CAD build for the part. Positions are in the model's coordinates, mm. A direction names the side the tool comes from. Give positions to 0.01 mm unless a question says otherwise; leave off trailing zeros. Write each loop counter-clockwise with the first axis right and the second up, starting at its lowest first coordinate (ties: lowest second). Pieces come first, ordered by that corner, then holes. Notation, with made-up numbers: (44, -31) - (62, -31) arc R21 ccw to (62, -15) - close; hole circle Ø1 at (66.5, 24). An arc over 180 degrees is marked (long way). Answer as a JSON object with one key per item and string values.
from build123d import *

# Parameters (mm, degrees)
SKETCH_1_W          = 41
SKETCH_1_H          = 64
EXTRUDE_1_DEPTH     = 4
SKETCH_2_R          = 1.75
CUT_EXTRUDE_1_DEPTH = 3
FILLET_1_R          = 2
CHAMFER_2_SIZE      = 1
CHAMFER_1_SIZE      = 2
CHAMFER_3_SIZE      = 0.5


with BuildPart() as part:
    # Эскиз1 → Бобышка-Вытянуть1 (new body)
    with BuildSketch(Plane(origin=(0, 0, 0), x_dir=(1, 0, 0), z_dir=(0, 1, 0))):
        Rectangle(SKETCH_1_W, SKETCH_1_H)
    extrude(amount=EXTRUDE_1_DEPTH)

    # Эскиз2 → Вырез-Вытянуть1 (cut)
    with BuildSketch(Plane(origin=(0, 4, 0), x_dir=(1, 0, 0), z_dir=(0, 1, 0))):
        with Locations(Location((16, 18, 0), (0, 0, 270))):
            Circle(SKETCH_2_R)
        with Locations(Location((16, -28, 0), (0, 0, 90))):
            Circle(SKETCH_2_R)
        with Locations(Location((-16, 18, 0), (0, 0, 90))):
            Circle(SKETCH_2_R)
        with Locations(Location((-16, -28, 0), (0, 0, 270))):
            Circle(SKETCH_2_R)
    extrude(amount=-CUT_EXTRUDE_1_DEPTH, mode=Mode.SUBTRACT)

    # Скругление1
    fillet_1_edges = [part.edges().sort_by_distance(p)[0] for p in [
        (20.5, 2, 32),
        (-20.5, 2, 32),
        (-20.5, 2, -32),
        (20.5, 2, -32),
    ]]
    fillet(fillet_1_edges, radius=FILLET_1_R)

    # Фаска2
    chamfer_2_edges = [part.edges().sort_by_distance(p)[0] for p in [
        (0, 4, -32),
        (20.5, 4, 0),
        (-20.5, 4, 0),
        (0, 4, 32),
        (19.914213562, 4, 31.414213562),
        (-19.914213562, 4, 31.414213562),
        (-19.914213562, 4, -31.414213562),
        (19.914213562, 4, -31.414213562),
    ]]
    chamfer(chamfer_2_edges, length=CHAMFER_2_SIZE)

    # Фаска1
    # the kernel refuses this chamfer: 2 mm, written as the material it takes off along each edge
    with BuildSketch(Plane(origin=(-16, 4, -18), x_dir=(0, 0, -1), z_dir=(1, 0, 0))) as chamfer_1_piece_1:
        Polygon((1.75 + CHAMFER_1_SIZE, 0), (1.75, -CHAMFER_1_SIZE), (1.75, 0), align=None)
    revolve(axis=Axis((-16, 4, -18), (0, 1, 0)), mode=Mode.SUBTRACT)
    with BuildSketch(Plane(origin=(-16, 4, 28), x_dir=(0, 0, 1), z_dir=(-1, 0, 0))) as chamfer_1_piece_2:
        Polygon((1.75 + CHAMFER_1_SIZE, 0), (1.75, -CHAMFER_1_SIZE), (1.75, 0), align=None)
    revolve(axis=Axis((-16, 4, 28), (0, 1, 0)), mode=Mode.SUBTRACT)
    with BuildSketch(Plane(origin=(16, 4, 28), x_dir=(0, 0, -1), z_dir=(1, 0, 0))) as chamfer_1_piece_3:
        Polygon((1.75 + CHAMFER_1_SIZE, 0), (1.75, -CHAMFER_1_SIZE), (1.75, 0), align=None)
    revolve(axis=Axis((16, 4, 28), (0, 1, 0)), mode=Mode.SUBTRACT)
    with BuildSketch(Plane(origin=(16, 4, -18), x_dir=(0, 0, 1), z_dir=(-1, 0, 0))) as chamfer_1_piece_4:
        Polygon((1.75 + CHAMFER_1_SIZE, 0), (1.75, -CHAMFER_1_SIZE), (1.75, 0), align=None)
    revolve(axis=Axis((16, 4, -18), (0, 1, 0)), mode=Mode.SUBTRACT)

    # Фаска3
    chamfer_3_edges = [part.edges().sort_by_distance(p)[0] for p in [
        (0, 0, -32),
        (20.5, 0, 0),
        (0, 0, 32),
        (-20.5, 0, 0),
        (19.914213562, 0, 31.414213562),
        (-19.914213562, 0, 31.414213562),
        (-19.914213562, 0, -31.414213562),
        (19.914213562, 0, -31.414213562),
    ]]
    chamfer(chamfer_3_edges, length=CHAMFER_3_SIZE)


solid = part.part
(1) Saw through at A-A, the plane x = 16. Give the cut face in (y, z) (3 decimals), and give its area (3 significant figures).
Answer key:
{"outline": "(0, -31.5) - (0.5, -32) - (3, -32) - (4, -31) - (4, -21.75) - (2, -19.75) - (1, -19.75) - (1, -16.25) - (2, -16.25) - (4, -14.25) - (4, 24.25) - (2, 26.25) - (1, 26.25) - (1, 29.75) - (2, 29.75) - (3.625, 31.375) - (3, 32) - (0.5, 32) - (0, 31.5) - close", "area": "226 mm²"}
(2) Pull direction X, two halves, no side cores. Call faces 3 (the face through (16, 1, 28)), 4 (the face through (0, 0, 0)), 5 (the face through (-20.5, 2, 0)), 6 (the face through (14.82, 1.51, 29.29)): pulls with the +X half, pulls with the -X half, needs draft (parallel to the pull), parting line crosses it, or undercut.
Answer key:
{"face 3": "undercut", "face 4": "needs draft", "face 5": "pulls with the -X half", "face 6": "undercut"}
(3) Probe L1, parallel to X at y = 1.8, z = -18; L2, parallel to Z at x = 18, y = 2.9; L3, parallel to Z at x = -16, y = 2.1. List the from-to ranges inside material, lowest first. Write a range as [from, to].
Answer key:
{"L1": "x = [-20.5, -17.75], [-14.25, 14.25], [17.75, 20.5]", "L2": "z = [-32, -19.74], [-16.26, 26.26], [29.74, 32]", "L3": "z = [-32, -19.85], [-16.15, 26.15], [29.85, 32]"}
(4) Flat gauge pins, fed straight in: P1, Ø4, axis at x = -16.5, z = -18, coming from the +Y side; P2, Ø4, axis at x = -16, z = -18, coming from the +Y side; P3, Ø1, axis at x = 16, z = 28, coming from the +Y side. Where does each tip first touch, or does it go through?
Answer key:
{"P1": "stops at y = 2.75", "P2": "stops at y = 2.25", "P3": "stops at y = 1"}
(5) 3-axis set-ups, long thin cutter, end or side, ignore diameter. For faces 1 (the face through (-19.1, 4, 30.4)), 2 (the face through (-17.735, 1.507, -17.772)): which of +Z, -Z, +X, -X, +Y, -Y reach the whole face in a straight line?
Answer key:
{"face 1": "+Z, -Z, +X, -X, +Y", "face 2": "+Y"}
(6) Saw through at B-B, the plane z = 28. Give the cut face in (x, y) (3 decimals), and give its area (3 significant figures).
Answer key:
{"outline": "(-20.5, 0.5) - (-20, 0) - (20, 0) - (20.5, 0.5) - (20.5, 3) - (19.625, 3.875) - (17.75, 2) - (17.75, 1) - (14.25, 1) - (14.25, 2) - (12.25, 4) - (-12.25, 4) - (-14.25, 2) - (-14.25, 1) - (-17.75, 1) - (-17.75, 2) - (-19.625, 3.875) - (-20.5, 3) - close", "area": "134 mm²"}
